Can you work these out from the model? Positions are in its coordinate system, mm. A direction names the side the tool comes from. Give positions to 0.01 mm unless a question says otherwise; leave off trailing zeros. Write each loop counter-clockwise with the first axis right and the second up, starting at its lowest first coordinate (ties: lowest second). Pieces come first, ordered by that corner, then holes. Notation, with made-up numbers: (32, 22) -> (79, 22) arc R18 cw to (79, 38) -> close; hole circle Ø11 at (-23.75, 29.25). An arc over 180 degrees is marked (long way). One line per item, written item: value.
from build123d import *

# Parameters (mm, degrees)
F0_W     = 115
F0_H     = 35
F0_R     = 1.6
F0_R_2   = 5.05
F0_R_3   = 6
F1_DEPTH = 3
F3_DEPTH = 3
F5_DEPTH = 3
F7_DEPTH = 112
F8_R     = 2.1
F9_DEPTH = 4.2023227536


with BuildPart() as f1:
    # F0 (on Front) → F1 (new body)
    with BuildSketch(Plane.XZ):
        with Locations((-2.2430759668, 17.5)):
            Rectangle(F0_W, F0_H)
        with Locations((-44.7430759668, 19)):
            Circle(F0_R, mode=Mode.SUBTRACT)
        with Locations((-25, 19)):
            Circle(F0_R_2, mode=Mode.SUBTRACT)
        with Locations((0, 19)):
            Circle(F0_R_3, mode=Mode.SUBTRACT)
        with Locations((25, 19)):
            Circle(F0_R_2, mode=Mode.SUBTRACT)
        with Locations((40.2569240332, 19)):
            Circle(F0_R, mode=Mode.SUBTRACT)
    extrude(amount=F1_DEPTH)

    # F2 (on face) → F3 (join)
    with BuildSketch(Plane(origin=(-59.7430759668, 0, 0), x_dir=(0, -1, 0), z_dir=(-1, 0, 0))):
        Polygon((0, 0), (0, 35), (-17.954993993, 2.8193253092), align=None)
    extrude(amount=-F3_DEPTH)

    # F4 (on face) → F5 (join)
    with BuildSketch(Plane.YZ.offset(55.2569240332)):
        Polygon((18.0769208819, 2.9807693791), (0, 35), (0, 0), align=None)
    extrude(amount=-F5_DEPTH)

    # F6 (on face) → F7 (join)
    with BuildSketch(Plane(origin=(52.2569240332, 0, 0), x_dir=(0, -1, 0), z_dir=(-1, 0, 0))):
        Polygon((-17.4172232201, 4.1492765441), (-18.0769208819, 2.9807693791), (0, 0), (0, 1.2772871172), align=None)
    extrude(amount=F7_DEPTH)

    # F8 (on face) → F9 (cut, through all)
    with BuildSketch(Plane(origin=(0, -0.2050414688, 1.243477082), x_dir=(1, 0, 0), z_dir=(0, -0.1626966256, 0.9866761414))):
        with Locations((40.5074283481, 11.60009671)):
            Circle(F8_R)
        with Locations((-44.4925716519, 11.60009671)):
            Circle(F8_R)
    extrude(amount=-F9_DEPTH, mode=Mode.SUBTRACT)


solid = f1.part
1) Will these pins go through, and if not, where does the flat tip stop? pin 1 (4 mm diameter, centred on x = 40.26, z = 19, fed in from +Y); pin 2 (12 mm diameter, centred on x = 10.5, y = 7, fed in from -Z); pin 3 (5 mm diameter, centred on y = 11, z = 22.5, fed in from -X).
Answer list:
pin 1: stops at y = 0
pin 2: stops at z = 0.16
pin 3: passes through
2) If we section it at B-B (z = 19): Write out the boundary of the cut face in (x, y).
Answer list:
outline: (-59.74, -3) -> (-46.34, -3) -> (-46.34, 0) -> (-56.74, 0) -> (-56.74, 8.93) -> (-59.74, 8.93) -> close; (-43.14, -3) -> (-30.05, -3) -> (-30.05, 0) -> (-43.14, 0) -> close; (-19.95, -3) -> (-6, -3) -> (-6, 0) -> (-19.95, 0) -> close; (6, -3) -> (19.95, -3) -> (19.95, 0) -> (6, 0) -> close; (30.05, -3) -> (38.66, -3) -> (38.66, 0) -> (30.05, 0) -> close; (41.86, -3) -> (55.26, -3) -> (55.26, 9.03) -> (52.26, 9.03) -> (52.26, 0) -> (41.86, 0) -> close
3) We'd pull the mould along X, two halves only. Please class faces 4 (the face through (-58.26, 9.1, 1.43)), 5 (the face through (-6, -1, 19)), 6 (the face through (52.257, 5, 15)), 7 (the face through (55.257, 5, 14)): released by +X, released by -X, zero draft, split by the parting line, or undercut.
Answer list:
face 4: zero draft
face 5: undercut
face 6: undercut
face 7: released by +X
4) I need wall thicknesses on L1, parallel to Z at x = -25, y = -1.9; L2, parallel to X at y = 13.75, z = 10; L3, parallel to Y at x = -30, z = 17. Which ranges of each line are inside material? Lowest first, please.
Answer list:
L1: z = 0 to 13.95, 24.05 to 35
L2: x = -59.74 to -56.74, 52.26 to 55.26
L3: y = -3 to 0
5) If we section it at C-C (x = -48): Write out the boundary of the cut face in (y, z).
Answer list:
outline: (-3, 0) -> (0, 0) -> (18.08, 2.98) -> (17.42, 4.15) -> (0, 1.28) -> (0, 35) -> (-3, 35) -> close
6) If we section it at D-D (x = 25): Write out the boundary of the cut face in (y, z).
Answer list:
outline: (-3, 0) -> (0, 0) -> (18.08, 2.98) -> (17.42, 4.15) -> (0, 1.28) -> (0, 13.95) -> (-3, 13.95) -> close; (-3, 24.05) -> (0, 24.05) -> (0, 35) -> (-3, 35) -> close
7) If we section it at A-A (x = 0): Write out the boundary of the cut face in (y, z), and give its area (3 significant figures).
Answer list:
outline: (-3, 0) -> (0, 0) -> (18.08, 2.98) -> (17.42, 4.15) -> (0, 1.28) -> (0, 13) -> (-3, 13) -> close; (-3, 25) -> (0, 25) -> (0, 35) -> (-3, 35) -> close
area: 91.7 mm^2
8) For faces 1 (the face through (-2.959, 8.587, 2.693)), 2 (the face through (-58.26, 8.49, 19.78)), 3 (the face through (-44.95, 9.32, 2.18)), which set-ups out of +Z, -Z, +X, -X, +Y, -Y let a thin tool reach every point of the face, with its end or its side?
Answer list:
face 1: +Z
face 2: +Z, -X, +Y
face 3: none
